Check sheet for the modelled part. Datum: model origin and axes. Units: mm. Give positions to 0.01 mm unless a question says otherwise; leave off trailing zeros. Order: outer loops, then holes, each group sorted by start corner. A loop starts at its lowest first (then second) coordinate and runs counter-clockwise, first axis right, second up. Notation, with made-up numbers: (14, -10) - (23, -10) arc R22 ccw to (23, 25) - close; hole circle Ø10 at (25, 11). An arc over 180 degrees is marked (long way). Answer in a Markdown table with one row per item.
from build123d import *

# Parameters (mm, degrees)
FILLET1_R     = 1.27
FILLET2_R     = 0.254
CHAMFER1_SIZE = 1.27


with BuildPart() as part:
    # Sketch1 → Revolve1 (revolve)
    with BuildSketch(Plane.XY, mode=Mode.PRIVATE) as revolve1_sk:
        Polygon((0, 0), (0, 63.5), (-98.3869, 63.5), (-98.3869, 45.2374), (-94.107, 45.2374), (-94.107, 38.1), (-98.3869, 38.1), (-98.3869, 6.551201717), (-98.3869, 0), align=None)
    revolve(revolve1_sk.sketch.rotate(Axis((0, 0, 0), (0, 1, 0)), 270), axis=Axis((0, 0, 0), (0, 1, 0)))

    # Fillet1
    fillet1_edges = [part.edges().sort_by_distance(p)[0] for p in [
        (0, 38.1, 94.107),
        (0, 45.2374, 94.107),
    ]]
    fillet(fillet1_edges, radius=FILLET1_R)

    # Fillet2
    fillet2_edges = [part.edges().sort_by_distance(p)[0] for p in [
        (0, 38.1, 98.3869),
        (0, 45.2374, 98.3869),
    ]]
    fillet(fillet2_edges, radius=FILLET2_R)

    # Chamfer1
    chamfer1_edges = [part.edges().sort_by_distance(p)[0] for p in [
        (0, 0, 98.3869),
    ]]
    chamfer(chamfer1_edges, length=CHAMFER1_SIZE)

    # Sketch7 → 3/8 NPT Tapped Hole3 (revolve, cut)
    with BuildSketch(Plane(origin=(0, 0, 0), x_dir=(0, 0, -1), z_dir=(1, 0, 0))):
        Polygon((0, 0), (0, 63.5), (7.1374, 63.5), (7.1374, 10.3378), (8.250003024, 10.3378), (8.5727413, 0), align=None)
    revolve(axis=Axis((0, -6.35, 0), (0, 1, 0)), mode=Mode.SUBTRACT)


solid = part.part
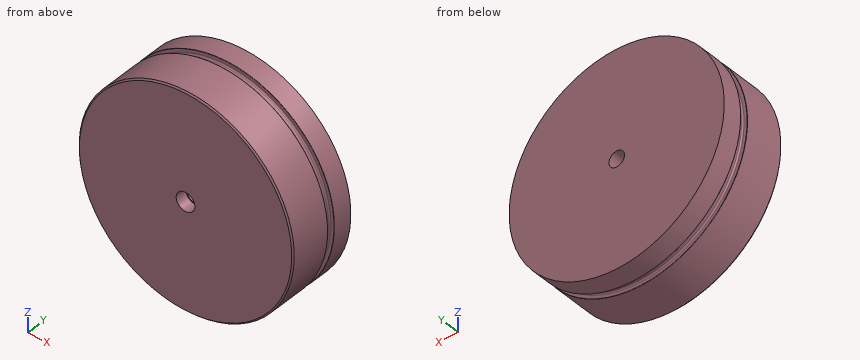
(1) Gauge pin test, flat ends, axial feed: P1, Ø12, axis at x = -76.5, z = -21.5, coming from the -Y side; P2, Ø10, axis at y = 6.5, z = -57.5, coming from the +X side; P3, Ø3, axis at x = -75.5, y = 14, coming from the +Z side; P4, Ø3, axis at y = 47, z = 78, coming from the -X side. Record the tip position at first contact, or that the pin passes through.
Geometry says:
| item | result |
|---|---|
| P1 | y = 0 |
| P2 | x = 83.21 |
| P3 | z = 64.84 |
| P4 | x = -61.87 |
(2) Cross-section at C-C, the plane y = 18. Record the cut outline in (x, z), then the cut area to 3 significant figures.
Geometry says:
| item | result |
|---|---|
| outline | circle Ø196.77 at (0, 0); hole circle Ø14.27 at (0, 0) |
| area | 30,300 mm² |
(3) Thickness scan on L1, parallel to X at y = 22, z = 0; L2, parallel to X at y = 44, z = 0; L3, parallel to Z at x = -83.5, y = 60.5. Record the ranges inside material, lowest first.
Geometry says:
| item | result |
|---|---|
| L1 | -98.39 to -7.14, 7.14 to 98.39 |
| L2 | -94.11 to -7.14, 7.14 to 94.11 |
| L3 | -52.04 to 52.04 |
